```python
from build123d import *

# Parameters (mm, degrees)
F1_DEPTH = 10.25
F2_T     = -1.9
F4_DEPTH = 2.25
F5_R     = 1


with BuildPart() as f1:
    # F0 (on Top) → F1 (new body)
    with BuildSketch(Plane.XY):
        with BuildLine():
            Line((16, 19), (-16, 19))
            ThreePointArc((-16, 19), (-21.6568542495, 16.6568542495), (-24, 11))
            Line((-24, 11), (-24, -11))
            ThreePointArc((-24, -11), (-21.6568542495, -16.6568542495), (-16, -19))
            Line((-16, -19), (16, -19))
            ThreePointArc((16, -19), (21.6568542495, -16.6568542495), (24, -11))
            Line((24, -11), (24, 11))
            ThreePointArc((24, 11), (21.6568542495, 16.6568542495), (16, 19))
        make_face()
    extrude(amount=F1_DEPTH)

    # F2
    f2_openings = [f1.faces().sort_by_distance(p)[0] for p in [
        (0, 0, 0),
    ]]
    offset(amount=F2_T, openings=f2_openings)

    # F3 (on face) → F4 (join)
    with BuildSketch(Plane.XY.offset(10.25)):
        with BuildLine():
            Line((12, 21.85), (-16, 21.85))
            ThreePointArc((-16, 21.85), (-21.6568542495, 19.5068542495), (-24, 13.85))
            Line((-24, 13.85), (-24, 11))
            ThreePointArc((-24, 11), (-21.6568542495, 16.6568542495), (-16, 19))
            Line((-16, 19), (12, 19))
            Line((12, 19), (12, 21.85))
        make_face()
        with BuildLine():
            Line((12, -21.85), (12, -19))
            Line((12, -19), (-16, -19))
            ThreePointArc((-16, -19), (-21.6568542495, -16.6568542495), (-24, -11))
            Line((-24, -11), (-24, -13.85))
            ThreePointArc((-24, -13.85), (-21.6568542495, -19.5068542495), (-16, -21.85))
            Line((-16, -21.85), (12, -21.85))
        make_face()
    extrude(amount=-F4_DEPTH)

    # F5
    f5_edges = [f1.edges().sort_by_distance(p)[0] for p in [
        (12, 19, 9.125),
        (12, 21.85, 9.125),
        (12, -19, 9.125),
        (12, -21.85, 9.125),
    ]]
    fillet(f5_edges, radius=F5_R)


solid = f1.part
```
Read the model definition and answer for the solid it produces. Units are mm, in the model's axes. A direction names the side the tool comes from. Round coordinates to 2 decimals unless told otherwise and drop trailing zeros. Write each loop counter-clockwise with the first axis right and the second up, starting at its lowest first coordinate (ties: lowest second). Pieces come first, ordered by that corner, then holes. Notation, with made-up numbers: M 74.5,33 L 107.5,33 A17 ccw 107.5,47 Z; hole C 29.25,30 d2. An arc over 180 degrees is marked long. One line per item, written item: value.
Q1. Flat-ended cylindrical pins translate along their axes: pin 1 Ø4 at (x, y) = (-12.5, -17) entering from -Z; pin 2 Ø0.7 at (y, z) = (-20.5, 9) entering from +X; pin 3 Ø1.5 at (y, z) = (-16.5, 8.5) entering from -X; pin 4 Ø6 at (x, z) = (-11.5, 2) entering from +Y. Find the tip coordinate at first contact, or state that the pin passes through.
Data:
pin 1: z = 0
pin 2: x = 12
pin 3: x = -23.77
pin 4: y = 19
Q2. Straight lines are drawn through the part: line 1 (Y direction, x = -8.5, z = 2.5); line 2 (X direction, y = 10.5, z = 2.75); line 3 (Z direction, x = 10.5, y = -9). For each, find the intervals that lie inside material, in ascending order. Write a range as [from, to].
Data:
line 1: [-19, -17.1], [17.1, 19]
line 2: [-24, -22.1], [22.1, 24]
line 3: [8.35, 10.25]
Q3. Find section B-B on y = -1. Write down the section's boundary in (x, z), plus the area to 3 significant figures.
Data:
outline: M -24,0 L -22.1,0 L -22.1,8.35 L 22.1,8.35 L 22.1,0 L 24,0 L 24,10.25 L -24,10.25 Z
area: 123 mm2
Q4. Find section D-D on y = -12. Write down the section's boundary in (x, z).
Data:
outline: M -24,8 L -23.94,8 L -23.94,0 L -22.02,0 L -22.02,8.35 L 22.02,8.35 L 22.02,0 L 23.94,0 L 23.94,10.25 L -24,10.25 Z
Q5. Find section C-C on x = 3. Write down the section's boundary in (y, z), plus the area to 3 significant figures.
Data:
outline: M -21.85,8 L -19,8 L -19,0 L -17.1,0 L -17.1,8.35 L 17.1,8.35 L 17.1,0 L 19,0 L 19,8 L 21.85,8 L 21.85,10.25 L -21.85,10.25 Z
area: 117 mm2
Q6. For a pull along X with two mould halves and no side action, classify faces 4 (the cylindrical face through (-20.361, -15.266, 4.117)), 5 (the flat face through (22.1, 0, 4)), 6 (the cylindrical face through (11.699, 21.565, 9.109)), 7 (the flat face through (-7, 20, 8)) as +X half, -X half, draft (parallel to the pull), parting line (faces both ways), or undercut.
Data:
face 4: undercut
face 5: undercut
face 6: +X half
face 7: draft
Q7. Find section A-A on z = 6.75. Write down the section's boundary in (x, y), plus the area to 3 significant figures.
Data:
outline: M -24,-11 A8 ccw -16,-19 L 16,-19 A8 ccw 24,-11 L 24,11 A8 ccw 16,19 L -16,19 A8 ccw -24,11 Z; hole M -22.1,-11 A6.1 ccw -16,-17.1 L 16,-17.1 A6.1 ccw 22.1,-11 L 22.1,11 A6.1 ccw 16,17.1 L -16,17.1 A6.1 ccw -22.1,11 Z
area: 289 mm2
Q8. Which of the six approach directions +Z, -Z, +X, -X, +Y, -Y give full straight-line access (tool end or side, diameter ignored) to faces 1 (the flat face through (0, 0, 8.35)), 2 (the flat face through (-6, -20, 8)), 3 (the cylindrical face through (-21.594, 16.719, 3.944))?
Data:
face 1: -Z
face 2: -Z, -X, -Y
face 3: -Z, -X, +Y
